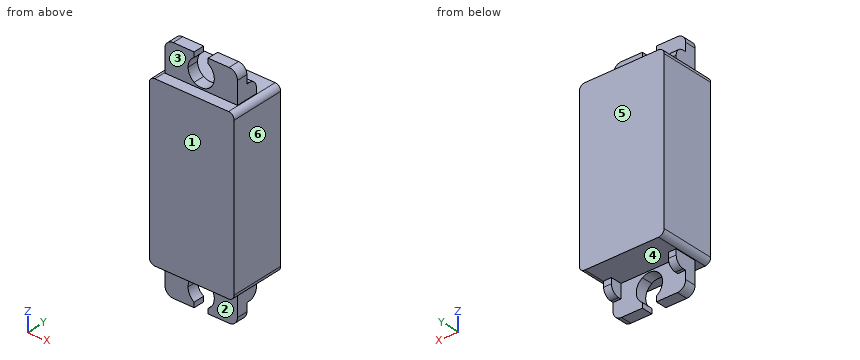
```python
from build123d import *

# Parameters (mm, degrees)
SKETCH1_W            = 15.2
SKETCH1_H            = 30.1
BOSS_EXTRUDE1_DEPTH  = 9.85
SKETCH2_W            = 13
SKETCH2_H            = 2
BOSS_EXTRUDE2_DEPTH  = 5.5
CUT_EXTRUDE2_DEPTH   = 23.677852632
FILLET1_R            = 1.5
SKETCH4_W            = 1.4
SKETCH4_H            = 2.5
BOSS_EXTRUDE3_DEPTH  = 2
FILLET3_R            = 1.5
FILLET3_OF_MIRROR1_R = 1.5
FILLET4_R            = 1


# Read off the part's stored shape, not the designer's step: Mirror2
with BuildPart() as part:
    # Sketch1 → Boss-Extrude1 (new body)
    with BuildSketch(Plane(origin=(0, 0, 0), x_dir=(1, 0, 0), z_dir=(0, 1, 0))):
        Rectangle(SKETCH1_W, SKETCH1_H)
    extrude(amount=BOSS_EXTRUDE1_DEPTH)

    # Sketch2 → Boss-Extrude2 (add)
    with BuildSketch(Plane.XY.offset(15.05)):
        with Locations((0, 3)):
            Rectangle(SKETCH2_W, SKETCH2_H)
    extrude(amount=BOSS_EXTRUDE2_DEPTH)

    # Sketch3 → Cut-Extrude2 (cut, through all)
    with BuildSketch(Plane(origin=(0, 4, 0), x_dir=(-1, 0, 0), z_dir=(0, 1, 0))):
        with BuildLine():
            Line((-1.25, 15.663025126), (-1.25, 17.653))
            Line((-1.25, 17.653), (-1.25, 19.642974874))
            ThreePointArc((-1.25, 19.642974874), (-2.35, 17.653), (-1.25, 15.663025126))
        make_face()
        with BuildLine():
            Line((-1.25, 19.642974874), (-1.25, 17.653))
            Line((-1.25, 17.653), (1.25, 17.653))
            Line((1.25, 17.653), (1.25, 19.642974874))
            ThreePointArc((1.25, 19.642974874), (0, 20.003), (-1.25, 19.642974874))
        make_face()
        with BuildLine():
            Line((1.25, 17.653), (-1.25, 17.653))
            Line((-1.25, 17.653), (-1.25, 15.663025126))
            ThreePointArc((-1.25, 15.663025126), (0, 15.303), (1.25, 15.663025126))
            Line((1.25, 15.663025126), (1.25, 17.653))
        make_face()
        with BuildLine():
            Line((1.25, 19.642974874), (1.25, 17.653))
            Line((1.25, 17.653), (1.25, 15.663025126))
            ThreePointArc((1.25, 15.663025126), (2.05669638, 16.5161183), (2.35, 17.653))
            ThreePointArc((2.35, 17.653), (2.05669638, 18.7898817), (1.25, 19.642974874))
        make_face()
        with BuildLine():
            Line((-1.25, 20.55), (-1.25, 19.642974874))
            ThreePointArc((-1.25, 19.642974874), (0, 20.003), (1.25, 19.642974874))
            Line((1.25, 19.642974874), (1.25, 20.55))
            Line((1.25, 20.55), (-1.25, 20.55))
        make_face()
    extrude(amount=-CUT_EXTRUDE2_DEPTH, mode=Mode.SUBTRACT)

    # Fillet1
    fillet1_edges = [part.edges().sort_by_distance(p)[0] for p in [
        (6.5, 3, 20.55),
        (-6.5, 3, 20.55),
    ]]
    fillet(fillet1_edges, radius=FILLET1_R)

    # Sketch4 → Boss-Extrude3 (add)
    with BuildSketch(Plane(origin=(0, 4, 0), x_dir=(-1, 0, 0), z_dir=(0, 1, 0))):
        with Locations((5.8, 16.3)):
            Rectangle(SKETCH4_W, SKETCH4_H)
    boss_extrude3 = extrude(amount=BOSS_EXTRUDE3_DEPTH)

    # Fillet3
    fillet3_edges = [part.edges().sort_by_distance(p)[0] for p in [
        (-5.8, 6, 17.55),
    ]]
    fillet(fillet3_edges, radius=FILLET3_R)

    # Mirror1: Boss-Extrude3 across plane
    add(boss_extrude3.mirror(Plane(origin=(0, 0, 0), x_dir=(0, 0, 1), z_dir=(1, 0, 0))))

    # Fillet3 of Mirror1
    fillet3_of_mirror1_edges = [part.edges().sort_by_distance(p)[0] for p in [
        (5.8, 6, 17.55),
    ]]
    fillet(fillet3_of_mirror1_edges, radius=FILLET3_OF_MIRROR1_R)

    # Mirror2: part across plane


with BuildPart() as part_1:
    add(part.part)
    add(part.part.mirror(Plane.XY))

    # Fillet4
    fillet4_edges = [part_1.edges().sort_by_distance(p)[0] for p in [
        (-7.6, 4.925, -15.05),
        (7.6, 4.925, -15.05),
        (7.6, 4.925, 15.05),
        (-7.6, 4.925, 15.05),
    ]]
    fillet(fillet4_edges, radius=FILLET4_R)


solid = part_1.part
```
Input: part model. Units: mm. Frame: model coordinates. Face numbers are marked on the shaded views. A direction names the side the tool comes from. Give positions to 0.01 mm unless a question says otherwise; leave off trailing zeros. Loops run counter-clockwise (first coordinate to the right, second up) from the corner with the lowest first, then second, coordinate; pieces in that order, holes last. Notation, with made-up numbers: (-27.5, 69.25) -> (6.5, 69.25) arc R14 ccw to (6.5, 95.25) -> close; hole circle Ø9 at (1, 56). An arc over 180 degrees is marked (long way). Use a Markdown table: item, result.
Q1. Pull-direction query (X, two-part tool) for the marked faces 4, 5 and 6; classes: pulls with the +X half, pulls with the -X half, needs draft (parallel to the pull), parting line crosses it, or undercut.
Entries:
| item | result |
|---|---|
| face 4 | undercut |
| face 5 | needs draft |
| face 6 | pulls with the +X half |
Q2. First-contact query: P1, Ø5, axis at y = 4.5, z = 14.5, coming from the +X side; P2, Ø1.6, axis at x = -0.5, z = 18, coming from the +Y side; P3, Ø3, axis at y = 5, z = 17.5, coming from the -X side; P4, Ø1.2, axis at y = 4, z = -17.5, coming from the +X side. Flat tips, straight axial feed; report the tip coordinate or a pass-through.
Entries:
| item | result |
|---|---|
| P1 | stops at x = 7.6 |
| P2 | passes through |
| P3 | stops at x = -6.5 |
| P4 | stops at x = 6.5 |
Q3. Ray query, probe 1 along Z at (x, y) = (-2, 9); probe 2 along X at (y, z) = (2.75, -17); probe 3 along Y at (x, z) = (5, 18). Return the intervals inside material, ascending. Write a range as from..to.
Entries:
| item | result |
|---|---|
| probe 1 | z = -15.05..15.05 |
| probe 2 | x = -6.5..-2.26, 2.26..6.5 |
| probe 3 | y = 2..4 |
Q4. Section query C-C, the plane x = 0. Return the cut outline in (y, z).
Entries:
| item | result |
|---|---|
| outline | (0, -15.05) -> (2, -15.05) -> (2, -15.3) -> (4, -15.3) -> (4, -15.05) -> (9.85, -15.05) -> (9.85, 15.05) -> (4, 15.05) -> (4, 15.3) -> (2, 15.3) -> (2, 15.05) -> (0, 15.05) -> close |
Q5. Section query A-A, the plane y = 6.5. Return the cut outline in (x, z).
Entries:
| item | result |
|---|---|
| outline | (-7.6, -14.05) arc R1 ccw to (-6.6, -15.05) -> (6.6, -15.05) arc R1 ccw to (7.6, -14.05) -> (7.6, 14.05) arc R1 ccw to (6.6, 15.05) -> (-6.6, 15.05) arc R1 ccw to (-7.6, 14.05) -> close |
Q6. Section query B-B, the plane z = 17. Return the cut outline in (x, y), plus the area to 3 significant figures.
Entries:
| item | result |
|---|---|
| outline | (-6.5, 2) -> (-2.26, 2) -> (-2.26, 4) -> (-5.1, 4) -> (-5.1, 5.66) -> (-6.5, 5.66) -> close; (2.26, 2) -> (6.5, 2) -> (6.5, 5.66) -> (5.1, 5.66) -> (5.1, 4) -> (2.26, 4) -> close |
| area | 21.6 mm² |
Q7. Access query for the marked faces 1, 2 and 3. Directions: +Z, -Z, +X, -X, +Y, -Y. A direction counts if a zero-diameter tool reaches every point of the face in a straight line with its end or side. Return the directions, or none.
Entries:
| item | result |
|---|---|
| face 1 | +Z, -Z, +X, -X, -Y |
| face 2 | -Z, +X, -X, -Y |
| face 3 | +Z, +X, -X, -Y |
